Here's how the part is built. I have some questions about the finished solid (model axes, mm). Face numbers are marked on the shaded views. A direction names the side the tool comes from. Round coordinates to 2 decimals unless told otherwise and drop trailing zeros. Order: outer loops, then holes, each group sorted by start corner. A loop starts at its lowest first (then second) coordinate and runs counter-clockwise, first axis right, second up.
```python
from build123d import *

# Parameters (mm, degrees)
SKETCH1_W                = 100
SKETCH1_H                = 45
BOSS_EXTRUDE1_DEPTH      = 2
BOSS_EXTRUDE2_DEPTH      = 100
BOSS_EXTRUDE3_DEPTH      = 15
CHAMFER2_SIZE            = 2
BOSS_EXTRUDE4_DEPTH      = 3
BOSS_EXTRUDE4_DEPTH_BACK = 48
SKETCH4_W                = 3
SKETCH4_H                = 35.5
BOSS_EXTRUDE6_DEPTH      = 103
CUT_EXTRUDE1_DEPTH       = 108
FILLET1_R                = 12
FILLET2_R                = 10


# Read off the part's stored shape, not the designer's step: Boss-Extrude6
with BuildPart() as part:
    # Sketch1 → Boss-Extrude1 (new body)
    with BuildSketch(Plane(origin=(0, 0, 0), x_dir=(1, 0, 0), z_dir=(0, 1, 0))):
        with Locations((50, 22.5)):
            Rectangle(SKETCH1_W, SKETCH1_H)
    extrude(amount=BOSS_EXTRUDE1_DEPTH)

    # Sketch2 → Boss-Extrude2 (add)
    with BuildSketch(Plane.ZY):
        Polygon((0, 2), (0, 22), (3, 22), (3, 0), (0, 0), align=None)
        Polygon((-45, 2), (-45, 22), (-48, 22), (-48, 0), (-45, 0), align=None)
    extrude(amount=-BOSS_EXTRUDE2_DEPTH)

    # Sketch3 → Boss-Extrude3 (add)
    with BuildSketch(Plane(origin=(100, 0, 0), x_dir=(0, 0, -1), z_dir=(1, 0, 0))):
        Polygon((0, 22), (0, 32.5), (45, 32.5), (45, 22), (48, 22), (48, 35.5), (-3, 35.5), (-3, 22), align=None)
    extrude(amount=-BOSS_EXTRUDE3_DEPTH)

    # Chamfer2
    chamfer2_edges = [part.edges().sort_by_distance(p)[0] for p in [
        (85, 32.5, -22.5),
    ]]
    chamfer(chamfer2_edges, length=CHAMFER2_SIZE)

    # Sketch4 → Boss-Extrude4 (add, two sides: drawn at the far end of the back side and taken through both)
    with BuildSketch(Plane.XY.offset(-BOSS_EXTRUDE4_DEPTH_BACK)):
        with Locations((101.5, 17.75)):
            Rectangle(SKETCH4_W, SKETCH4_H)
    extrude(amount=BOSS_EXTRUDE4_DEPTH + BOSS_EXTRUDE4_DEPTH_BACK)

    # Boss-Extrude6 outline → Boss-Extrude6 (add)
    with BuildSketch(Plane.YZ):
        with BuildLine():
            Line((0, -48), (0, -31.964101615))
            ThreePointArc((0, -31.964101615), (-0.068148347, -32.481739705), (-0.267949192, -32.964101615))
            Line((-0.267949192, -32.964101615), (-3.78757632, -39.060274624))
            ThreePointArc((-3.78757632, -39.060274624), (-4.037826078, -39.794785514), (-3.989674587, -40.569261223))
            Line((-3.989674587, -40.569261223), (-2.034217014, -48))
            Line((-2.034217014, -48), (0, -48))
        make_face()
        with BuildLine():
            ThreePointArc((-3.989674587, -4.430738777), (-4.037826078, -5.205214486), (-3.78757632, -5.939725376))
            Line((-3.78757632, -5.939725376), (-0.267949192, -12.035898385))
            ThreePointArc((-0.267949192, -12.035898385), (-0.068148347, -12.518260295), (0, -13.035898385))
            Line((0, -13.035898385), (0, 3))
            Line((0, 3), (-2.034217014, 3))
            Line((-2.034217014, 3), (-3.989674587, -4.430738777))
        make_face()
    extrude(amount=BOSS_EXTRUDE6_DEPTH)

    # Sketch6 → Cut-Extrude1 (cut)
    with BuildSketch(Plane.ZY):
        with BuildLine():
            Line((-39.060274624, -3.78757632), (-39.060274624, -2.38757632))
            ThreePointArc((-39.060274624, -2.38757632), (-39.323878521, -1.751180217), (-39.960274624, -1.48757632))
            Line((-39.960274624, -1.48757632), (-40.160274624, -1.48757632))
            ThreePointArc((-40.160274624, -1.48757632), (-40.796670727, -1.751180217), (-41.060274624, -2.38757632))
            Line((-41.060274624, -2.38757632), (-41.060274624, -3.860460534))
            Line((-41.060274624, -3.860460534), (-41.060274624, -4.910280297))
            Line((-41.060274624, -4.910280297), (-39.060274624, -4.910280297))
            Line((-39.060274624, -4.910280297), (-39.060274624, -3.78757632))
        make_face()
        with BuildLine():
            Line((-5.939725376, -3.78757632), (-5.939725376, -2.38757632))
            ThreePointArc((-5.939725376, -2.38757632), (-5.676121479, -1.751180217), (-5.039725376, -1.48757632))
            Line((-5.039725376, -1.48757632), (-4.839725376, -1.48757632))
            ThreePointArc((-4.839725376, -1.48757632), (-4.203329273, -1.751180217), (-3.939725376, -2.38757632))
            Line((-3.939725376, -2.38757632), (-3.939725376, -3.860460534))
            Line((-3.939725376, -3.860460534), (-3.939725376, -5.247114717))
            Line((-3.939725376, -5.247114717), (-5.939725376, -5.247114717))
            Line((-5.939725376, -5.247114717), (-5.939725376, -3.78757632))
        make_face()
    extrude(amount=-CUT_EXTRUDE1_DEPTH, mode=Mode.SUBTRACT)

    # Fillet1
    fillet1_edges = [part.edges().sort_by_distance(p)[0] for p in [
        (85, 22, 1.5),
        (85, 22, -46.5),
    ]]
    fillet(fillet1_edges, radius=FILLET1_R)

    # Fillet2
    fillet2_edges = [part.edges().sort_by_distance(p)[0] for p in [
        (0, 22, 1.5),
        (0, 22, -46.5),
    ]]
    fillet(fillet2_edges, radius=FILLET2_R)


solid = part.part
```
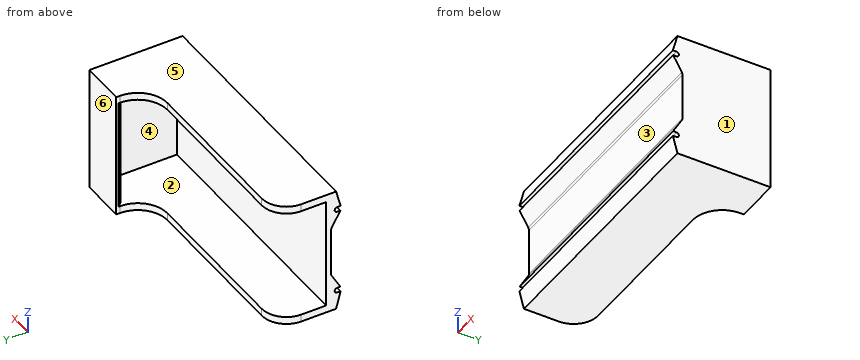
1. If we section it at A-A, the plane y = 7.5: Write out the boundary of the cut face in (x, z), and give its area (3 significant figures).
Evaluation:
outline: (0, -48) - (103, -48) - (103, 3) - (0, 3) - (0, 0) - (100, 0) - (100, -45) - (0, -45) - close
area: 753 mm2
2. I need wall thicknesses on probe 1 along Z at (x, y) = (83.5, 10.5); probe 2 along X at (y, z) = (25.5, -37); probe 3 along Z at (x, y) = (90, -1). Which ranges of each line are inside material? Lowest first, please.
Evaluation:
probe 1: z = -48 to -45, 0 to 3
probe 2: x = 100 to 103
probe 3: z = -48 to -34.23, -10.77 to 3
3. I'm going to push flat-ended pins straight in: P1, Ø2.5, axis at x = 46, z = 1.5, coming from the +Y side; P2, Ø1.5, axis at y = 17, z = -13.5, coming from the -X side; P3, Ø13.5, axis at x = 58, z = -18.5, coming from the +Y side. Where does each tip first touch, or does it pass through?
Evaluation:
P1: stops at y = 22
P2: stops at x = 100
P3: stops at y = 2
4. If we mould it in two halves opening along Z, with no side actions, what happens to the marked faces 4, 5 and 6? For each: released by +Z, released by -Z, zero draft, split by the parting line, or undercut.
Evaluation:
face 4: undercut
face 5: released by +Z
face 6: zero draft
5. On a 3-axis mill with a long thin cutter (end or side, diameter ignored), from which of +Z, -Z, +X, -X, +Y, -Y can I reach the whole of each face in a straight line? I mean the marked faces 1, 2 and 3. Say none if no direction works.
Evaluation:
face 1: +Z, -Z, +X, +Y, -Y
face 2: -X
face 3: +X, -X, -Y
6. If we section it at D-D, the plane y = 23: Write out the boundary of the cut face in (x, z).
Evaluation:
outline: (77.8, -48) - (103, -48) - (103, 3) - (77.8, 3) - (77.8, 0) - (100, 0) - (100, -45) - (77.8, -45) - close
7. If we section it at C-C, the plane x = 67.5: Write out the boundary of the cut face in (y, z).
Evaluation:
outline: (-3.86, -41.06) - (-2.03, -48) - (22, -48) - (22, -45) - (2, -45) - (2, 0) - (22, 0) - (22, 3) - (-2.03, 3) - (-3.86, -3.94) - (-2.39, -3.94) arc R0.9 cw to (-1.49, -4.84) - (-1.49, -5.04) arc R0.9 cw to (-2.39, -5.94) - (-3.79, -5.94) - (-0.27, -12.04) arc R2 cw to (0, -13.04) - (0, -31.96) arc R2 cw to (-0.27, -32.96) - (-3.79, -39.06) - (-2.39, -39.06) arc R0.9 cw to (-1.49, -39.96) - (-1.49, -40.16) arc R0.9 cw to (-2.39, -41.06) - close
8. If we section it at B-B, the plane z = -27: Write out the boundary of the cut face in (x, y), and give its area (4 significant figures).
Evaluation:
outline: (0, 0) - (103, 0) - (103, 35.5) - (85, 35.5) - (85, 34.5) - (87, 32.5) - (100, 32.5) - (100, 2) - (0, 2) - close
area: 349.5 mm2
